For this review, take the finished solid that the model builds, in its own axes (mm). Face numbers are marked on the shaded views. Round coordinates to 2 decimals unless told otherwise and drop trailing zeros. Order: outer loops, then holes, each group sorted by start corner. A loop starts at its lowest first (then second) coordinate and runs counter-clockwise, first axis right, second up. Notation, with made-up numbers: M 88,79 L 112,79 A25 ccw 112,94 Z; hole C -39.75,31.5 d7. An arc over 180 degrees is marked long. Answer as a JSON object with one key per item and string values.
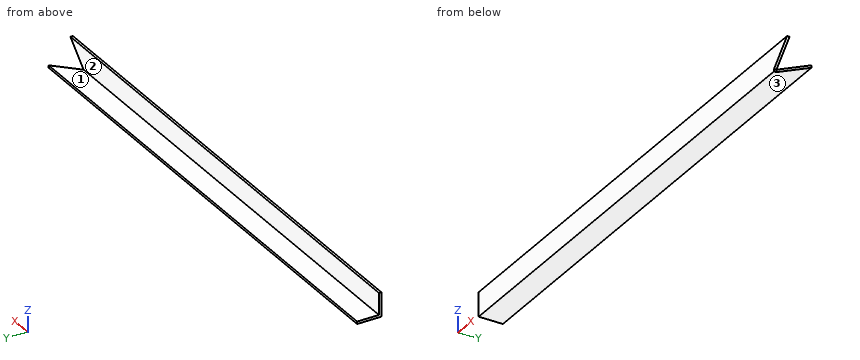
from build123d import *

# Parameters (mm, degrees)
F1_DEPTH = 1055
F4_DEPTH = 5
F5_DEPTH = 25
F6_DEPTH = 45


with BuildPart() as f1:
    # F0 (on Right) → F1 (new body)
    with BuildSketch(Plane.YZ):
        Polygon((0, 50), (0, 0), (50, 0), (50, 5), (5, 5), (5, 50), align=None)
    extrude(amount=F1_DEPTH)

    # F3 (on face) → F4 (cut)
    with BuildSketch(Plane.XY.offset(5)):
        Polygon((1055, 5), (1055, 50), (1010, 5), align=None)
    extrude(amount=-F4_DEPTH, mode=Mode.SUBTRACT)

    # F2 (on face) → F5 (cut)
    with BuildSketch(Plane(origin=(0, 5, 0), x_dir=(-1, 0, 0), z_dir=(0, 1, 0))):
        Polygon((-1055, 5), (-1010, 5), (-1055, 50), align=None)
    extrude(amount=-F5_DEPTH, mode=Mode.SUBTRACT)

    # F6 (cut): a face of the model
    f6_faces = [f1.faces().sort_by_distance(p)[0] for p in [
        (1055, 2.5, 2.5),
    ]]
    extrude(f6_faces, amount=-F6_DEPTH, mode=Mode.SUBTRACT)


solid = f1.part
1) Add section C-C on z = 28.5. State the section outline as (x, y) points.
Geometry check:
{"outline": "M 0,0 L 1033.5,0 L 1033.5,5 L 0,5 Z"}
2) For L1, parallel to Z at x = 560, y = 15.5, list the stretches that pass through material, from the lowest coordinate up.
Geometry check:
{"L1": "z = 0 to 5"}
3) Add section A-A on x = 322. State the section outline as (y, z) points, and give its area (3 significant figures).
Geometry check:
{"outline": "M 0,0 L 50,0 L 50,5 L 5,5 L 5,50 L 0,50 Z", "area": "475 mm²"}
4) Insertion check: P1, Ø2, axis at x = 194.5, y = 29.5, coming from the +Z side; P2, Ø2, axis at x = 770.5, z = 7, coming from the +Y side; P3, Ø1.5, axis at y = 3, z = 2, coming from the +X side; P4, Ø12, axis at y = 32, z = 16.5, coming from the +X side. Each pin has a flat end and moves straight along its axis. Give the tip position at first contact, or say it passes through.
Geometry check:
{"P1": "stops at z = 5", "P2": "stops at y = 5", "P3": "stops at x = 1010", "P4": "passes through"}
5) Mouldability with a two-part tool opening along Z and no side actions: class the marked faces 1, 2 and 3 as +Z half, -Z half, draft (parallel to the pull), parting line (faces both ways), or undercut.
Geometry check:
{"face 1": "+Z half", "face 2": "draft", "face 3": "-Z half"}
6) Add section B-B on y = 22. State the section outline as (x, z) points, and give its area (4 significant figures).
Geometry check:
{"outline": "M 0,0 L 1027,0 L 1027,5 L 0,5 Z", "area": "5,135 mm²"}
